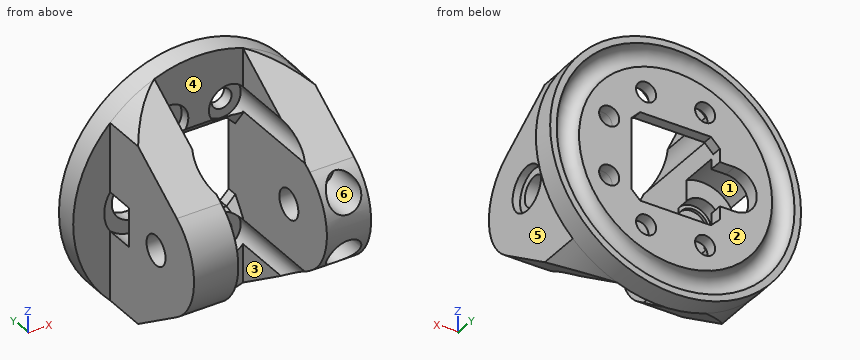
```python
from build123d import *

# Parameters (mm, degrees)
CUT_EXTRUDE1_DEPTH      = 5.7625
SKETCH4_R               = 7.62
CUT_EXTRUDE2_DEPTH      = 1.905
BOSS_EXTRUDE1_DEPTH     = 50.8
SKETCH6_R               = 3.175
CUT_EXTRUDE3_DEPTH      = 27.9875
CUT_EXTRUDE3_DEPTH_BACK = 27.9875
SKETCH7_R               = 7.62
CUT_EXTRUDE4_DEPTH      = 6.35
SKETCH8_R               = 3.96875
CUT_EXTRUDE5_DEPTH      = 2.7686
SKETCH9_R               = 3.2385
CUT_EXTRUDE6_DEPTH      = 0.635
CHAMFER1_SIZE           = 1.905
CHAMFER2_SIZE           = 2.54
SKETCH10_R              = 2.159
CUT_EXTRUDE7_DEPTH      = 3.38125
CUT_EXTRUDE7_DEPTH_BACK = 31.44825
CUT_EXTRUDE8_START      = -2.54
SKETCH11_R              = 4.1275
CUT_EXTRUDE8_DEPTH      = 31.2895001
CUT_EXTRUDE9_START      = -22.225
SKETCH12_R              = 3.556
CUT_EXTRUDE9_DEPTH      = 11.6045001
SKETCH13_R              = 4.7625
CUT_EXTRUDE10_DEPTH     = 1.6002


with BuildPart() as part:
    # Sketch2 → Revolve1 (revolve)
    with BuildSketch(Plane.XY):
        with BuildLine():
            Line((0, 0), (0, 2.38125))
            Line((0, 2.38125), (-20.767844423, 2.38125))
            ThreePointArc((-20.767844423, 2.38125), (-23.1775, 0.09525), (-25.587155577, 2.38125))
            Line((-25.587155577, 2.38125), (-26.9875, 2.38125))
            Line((-26.9875, 2.38125), (-26.9875, -2.38125))
            Line((-26.9875, -2.38125), (0, -2.38125))
            Line((0, -2.38125), (0, 0))
        make_face()
    revolve(axis=Axis((0, 0, 0), (0, 1, 0)))

    # Sketch3 → Cut-Extrude1 (cut, through all)
    with BuildSketch(Plane(origin=(0, 2.38125, 0), x_dir=(1, 0, 0), z_dir=(0, 1, 0))):
        with BuildLine():
            Line((-9.525, -9.525), (9.525, -9.525))
            Line((9.525, -9.525), (9.525, 9.525))
            Line((9.525, 9.525), (-9.525, 9.525))
            Line((-9.525, 9.525), (-9.525, 4.7625))
            Line((-9.525, 4.7625), (-12.7, 4.7625))
            ThreePointArc((-12.7, 4.7625), (-17.4625, 0), (-12.7, -4.7625))
            Line((-12.7, -4.7625), (-9.525, -4.7625))
            Line((-9.525, -4.7625), (-9.525, -9.525))
        make_face()
    extrude(amount=-CUT_EXTRUDE1_DEPTH, mode=Mode.SUBTRACT)

    # Sketch4 → Cut-Extrude2 (cut)
    with BuildSketch(Plane.XZ.offset(2.38125)):
        with Locations((-12.7, 0)):
            Circle(SKETCH4_R)
    extrude(amount=-CUT_EXTRUDE2_DEPTH, mode=Mode.SUBTRACT)

    # Sketch5 → Boss-Extrude1 (add)
    with BuildSketch(Plane.XZ.offset(2.38125)):
        with BuildLine():
            Line((-9.525, -25.250733281), (-9.525, 25.250733281))
            ThreePointArc((-9.525, 25.250733281), (-14.613052318, 22.688848763), (-19.05, 19.116031394))
            Line((-19.05, 19.116031394), (-19.05, -19.116031394))
            ThreePointArc((-19.05, -19.116031394), (-14.613052318, -22.688848763), (-9.525, -25.250733281))
        make_face()
        with BuildLine():
            Line((9.525, -25.250733281), (9.525, 25.250733281))
            ThreePointArc((9.525, 25.250733281), (14.613052318, 22.688848763), (19.05, 19.116031394))
            Line((19.05, 19.116031394), (19.05, -19.116031394))
            ThreePointArc((19.05, -19.116031394), (14.613052318, -22.688848763), (9.525, -25.250733281))
        make_face()
    extrude(amount=BOSS_EXTRUDE1_DEPTH)

    # Sketch6 → Cut-Extrude3 (cut, two sides)
    with BuildSketch(Plane(origin=(0, 0, 0), x_dir=(0, 0, -1), z_dir=(1, 0, 0))) as cut_extrude3_sk:
        with Locations((0, -17.74825)):
            Circle(SKETCH6_R)
        with BuildLine():
            Line((-25.250733281, -2.38125), (-25.250733281, -53.18125))
            Line((-25.250733281, -53.18125), (25.250733281, -53.18125))
            Line((25.250733281, -53.18125), (25.250733281, -2.38125))
            Line((25.250733281, -2.38125), (10.623124822, -24.708078951))
            ThreePointArc((10.623124822, -24.708078951), (0, -30.44825), (-10.623124822, -24.708078951))
            Line((-10.623124822, -24.708078951), (-25.250733281, -2.38125))
        make_face()
    extrude(amount=CUT_EXTRUDE3_DEPTH, mode=Mode.SUBTRACT)
    extrude(cut_extrude3_sk.sketch, amount=-CUT_EXTRUDE3_DEPTH_BACK, mode=Mode.SUBTRACT)

    # Sketch7 → Cut-Extrude4 (cut)
    with BuildSketch(Plane(origin=(0, -2.38125, 0), x_dir=(1, 0, 0), z_dir=(0, 1, 0))):
        with Locations((-12.7, 0)):
            Circle(SKETCH7_R)
    extrude(amount=-CUT_EXTRUDE4_DEPTH, mode=Mode.SUBTRACT)

    # Sketch8 → Cut-Extrude5 (cut)
    with BuildSketch(Plane(origin=(0, -8.73125, 0), x_dir=(1, 0, 0), z_dir=(0, 1, 0))):
        with Locations((-12.7, 0)):
            Circle(SKETCH8_R)
    extrude(amount=-CUT_EXTRUDE5_DEPTH, mode=Mode.SUBTRACT)

    # Sketch9 → Cut-Extrude6 (cut)
    with BuildSketch(Plane(origin=(0, -11.49985, 0), x_dir=(1, 0, 0), z_dir=(0, 1, 0))):
        with Locations((-12.7, 0)):
            Circle(SKETCH9_R)
    extrude(amount=-CUT_EXTRUDE6_DEPTH, mode=Mode.SUBTRACT)

    # Chamfer1
    chamfer1_edges = [part.edges().sort_by_distance(p)[0] for p in [
        (9.525, 0, -9.525),
        (9.525, 0, 9.525),
        (-9.525, 0, 9.525),
        (-9.525, 0, -9.525),
    ]]
    chamfer(chamfer1_edges, length=CHAMFER1_SIZE)

    # Chamfer2
    chamfer2_edges = [part.edges().sort_by_distance(p)[0] for p in [
        (0, -2.38125, 9.525),
        (0, -2.38125, -9.525),
        (-8.5725, -2.38125, 8.5725),
        (8.5725, -2.38125, 8.5725),
        (8.5725, -2.38125, -8.5725),
        (-8.5725, -2.38125, -8.5725),
    ]]
    chamfer(chamfer2_edges, length=CHAMFER2_SIZE)

    # Sketch10 → Cut-Extrude7 (cut, two sides)
    with BuildSketch(Plane(origin=(0, 0, 0), x_dir=(1, 0, 0), z_dir=(0, 1, 0))) as cut_extrude7_sk:
        with Locations((-6.35, 14.2875)):
            Circle(SKETCH10_R)
        with Locations((-6.35, -14.2875)):
            Circle(SKETCH10_R)
        with Locations((6.35, -14.2875)):
            Circle(SKETCH10_R)
        with Locations((6.35, 14.2875)):
            Circle(SKETCH10_R)
        with Locations((14.2875, 6.35)):
            Circle(SKETCH10_R)
        with Locations((14.2875, -6.35)):
            Circle(SKETCH10_R)
    extrude(amount=CUT_EXTRUDE7_DEPTH, mode=Mode.SUBTRACT)
    extrude(cut_extrude7_sk.sketch, amount=-CUT_EXTRUDE7_DEPTH_BACK, mode=Mode.SUBTRACT)

    # Sketch11 → Cut-Extrude8 (cut, through all)
    with BuildSketch(Plane(origin=(0, 2.38125, 0), x_dir=(1, 0, 0), z_dir=(0, 1, 0)).offset(CUT_EXTRUDE8_START)):
        with Locations((-6.35, 14.2875)):
            Circle(SKETCH11_R)
        with Locations((6.35, 14.2875)):
            Circle(SKETCH11_R)
        with Locations((6.35, -14.2875)):
            Circle(SKETCH11_R)
        with Locations((-6.35, -14.2875)):
            Circle(SKETCH11_R)
    extrude(amount=-CUT_EXTRUDE8_DEPTH, mode=Mode.SUBTRACT)

    # Sketch12 → Cut-Extrude9 (cut, through all)
    with BuildSketch(Plane(origin=(0, 2.38125, 0), x_dir=(1, 0, 0), z_dir=(0, 1, 0)).offset(CUT_EXTRUDE9_START)):
        with Locations((14.2875, 6.35)):
            Circle(SKETCH12_R)
        with Locations((14.2875, -6.35)):
            Circle(SKETCH12_R)
    extrude(amount=-CUT_EXTRUDE9_DEPTH, mode=Mode.SUBTRACT)

    # Sketch13 → Cut-Extrude10 (cut)
    with BuildSketch(Plane(origin=(19.05, 0, 0), x_dir=(0, 0, -1), z_dir=(1, 0, 0))):
        with Locations((0, -17.74825)):
            Circle(SKETCH13_R)
    extrude(amount=-CUT_EXTRUDE10_DEPTH, mode=Mode.SUBTRACT)


solid = part.part
```
Could you check a few things on this model? Use its own coordinates, in mm. Face numbers are marked on the shaded views. A direction names the side the tool comes from. Give positions to 0.01 mm unless a question says otherwise; leave off trailing zeros. Loops run counter-clockwise (first coordinate to the right, second up) from the corner with the lowest first, then second, coordinate; pieces in that order, holes last. Notation, with made-up numbers: (-3, 31.5) - (55, 31.5) arc R10 ccw to (55, 44.5) - close; hole circle Ø8 at (-28.75, 28.25). An arc over 180 degrees is marked (long way). Answer in a Markdown table with one row per item. Add a question column.
Q1. If we section it at A-A (x = 0): List the corners of the cut face in (y, z) for me (1 decimal).
Q2. We'd pull the mould along Y, two halves only. Please class the marked faces 1, 2 and 3: +Y half, -Y half, draft (parallel to the pull), parting line (faces both ways), or undercut.
Q3. Please list where these lines run through material, in increasing order: L1, parallel to X at y = -22, z = 6 (3 decimals); L2, parallel to Z at x = 13, y = -20; L3, parallel to X at y = -3, z = -5 (3 decimals). Write a range as from..to.
Q4. Which directions (+Z, -Z, +X, -X, +Y, -Y) give clear straight access to the entire face, cutting with the end or side of a thin tool? Please do the marked faces 4, 5 and 6.
Q5. For pin 1 (6.5 mm diameter, centred on x = -24, z = -8, fed in from -Y); pin 2 (1 mm diameter, centred on y = -14, z = -15.5, fed in from +X); pin 3 (6.5 mm diameter, centred on y = -7.5, z = -19.5, fed in from -X); pin 4 (9 mm diameter, centred on x = 14.29, z = -6.35, fed in from +Y), each with a flat end and sliding along its axis, tell me the tip position at first contact or that it passes through.
Q6. If we section it at C-C (y = -7): State how many separate pieces and enclosed holes the cut face has, plus the area to 3 significant figures.
The answers:
| question | item | result |
|---|---|---|
| 1 | outline | (-2.4, -27) - (2.4, -27) - (2.4, -25.6) arc R2.4 cw to (2.4, -20.8) - (2.4, -9.5) - (0.2, -9.5) - (-2.4, -12.1) - close; (-2.4, 12.1) - (0.2, 9.5) - (2.4, 9.5) - (2.4, 20.8) arc R2.4 cw to (2.4, 25.6) - (2.4, 27) - (-2.4, 27) - close |
| 2 | face 1 | undercut |
| 2 | face 2 | +Y half |
| 2 | face 3 | draft |
| 3 | L1 | x = -19.05..-9.525, 9.525..10.749, 17.826..19.05 |
| 3 | L2 | z = -13.71..-9.66, -3.04..-2.24, 2.24..3.04, 9.66..13.71 |
| 3 | L3 | x = -19.05..-18.45, 9.525..12.603, 15.972..19.05 |
| 4 | face 4 | +Z, -Z, -Y |
| 4 | face 5 | +Z, -Z, +X, -Y |
| 4 | face 6 | -Y |
| 5 | pin 1 | stops at y = -2.38 |
| 5 | pin 2 | stops at x = 19.05 |
| 5 | pin 3 | stops at x = -19.05 |
| 5 | pin 4 | stops at y = 2.38 |
| 6 | separate pieces | 3 |
| 6 | enclosed holes | 2 |
| 6 | area | 651 mm^2 |
